Can you work these out from the drawing? Everything is in mm from the part's minimum corner. Give positions to 0.01 mm unless a question says otherwise; leave off trailing zeros. Loops run counter-clockwise (first coordinate to the right, second up) from the corner with the lowest first, then second, coordinate; pieces in that order, holes last.
Q1. I need wall thicknesses on line 1 (Z direction, x = 6, y = 7); line 2 (Y direction, x = 5, z = 5.4); line 3 (Y direction, x = 33.5, z = 4.2). Which ranges of each line are inside material? Lowest first, please.
Q2. If we section it at B-B (y = 28): Please give me the cut outline in (x, z).
Q3. If we section it at A-A (z = 2.05): Please give me the cut outline in (x, y).
Q4. We'd pull the mould along Z, two halves only. Please class the marked faces 1, 2, 3 and 4: +Z half, -Z half, draft (parallel to the pull), parting line (faces both ways), or undercut.
Q5. If we section it at C-C (x = 31.5): Please give me the cut outline in (y, z), plus the area to 3 significant figures.
Q6. Will these pins go through, and if not, where does the flat tip stop? P1, Ø1.8, axis at y = 29.5, z = 4.5, coming from the -X side; P2, Ø1.2, axis at x = 31.5, z = 3, coming from the -Y side; P3, Ø1, axis at y = 25, z = 2.5, coming from the +X side; P4, Ø3, axis at y = 4.5, z = 4.5, coming from the +X side.
Q7. If we section it at D-D (y = 8): Please give me the cut outline in (x, z), plus the area to 3 significant figures.
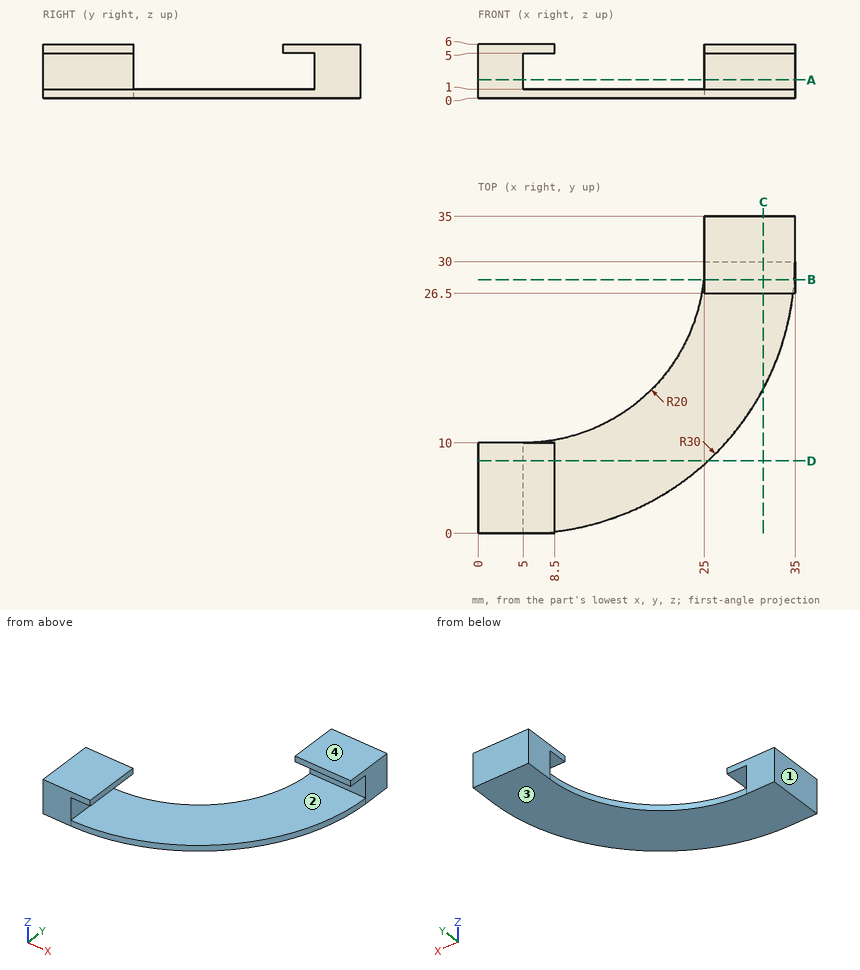
Check sheet entries:
1. line 1: z = 0 to 1, 5 to 6
1. line 2: y = 0 to 10
1. line 3: y = 30 to 35
2. outline: (24.9, 0) - (34.93, 0) - (34.93, 1) - (24.9, 1) - close; (25, 5) - (35, 5) - (35, 6) - (25, 6) - close
3. outline: (0, 0) - (5, 0) - (5, 10) - (0, 10) - close; (25, 30) - (35, 30) - (35, 35) - (25, 35) - close
4. face 1: draft
4. face 2: undercut
4. face 3: -Z half
4. face 4: +Z half
5. outline: (15.94, 0) - (35, 0) - (35, 6) - (26.5, 6) - (26.5, 5) - (30, 5) - (30, 1) - (15.94, 1) - close
5. area: 47.6 mm2
6. P1: stops at x = 25
6. P2: stops at y = 30
6. P3: passes through
6. P4: stops at x = 8.5
7. outline: (0, 0) - (25.4, 0) - (25.4, 1) - (5, 1) - (5, 5) - (8.5, 5) - (8.5, 6) - (0, 6) - close
7. area: 53.9 mm2
